Drawing for the job (mm, zero at the part's lowest x, y, z). Coordinates: 2 decimals unless noted, no trailing zeros. Order: outer loops, then holes, each group sorted by start corner. A loop starts at its lowest first (then second) coordinate and runs counter-clockwise, first axis right, second up. Notation, with made-up numbers: M -31.75,-36.5 L 16.25,-36.5 A26 ccw 16.25,-0.5 Z; hole C 54.5,17.25 d5. An arc over 180 degrees is marked long. Write item = value, one per line. Start each with the question number.
Q1. Band-saw the part on A-A on y = 7.5. Write the cut outline in (x, z), plus the area to 3 significant figures.
Q2. Drill centre lines: probe 1 along Y at (x, z) = (7.5, 1.35); probe 2 along Z at (x, y) = (13.25, 11.25); probe 3 along Y at (x, z) = (9, 3.75). Where is each one in solid material? Low to high.
Q3. Band-saw the part on C-C on z = 2.95. Write the cut outline in (x, y).
Q4. Pin check, flat tips, straight feed: P1, Ø1.5, axis at x = 6, z = 2, coming from the -Y side; P2, Ø2, axis at x = 9.5, z = 1.5, coming from the +Y side; P3, Ø2, axis at x = 12, z = 2.5, coming from the -Y side. Stop position of each tip, or through.
Q5. Pull direction X, two halves, no side cores. Call the marked faces 1, 2 and 3: released by +X, released by -X, zero draft, split by the parting line, or undercut.
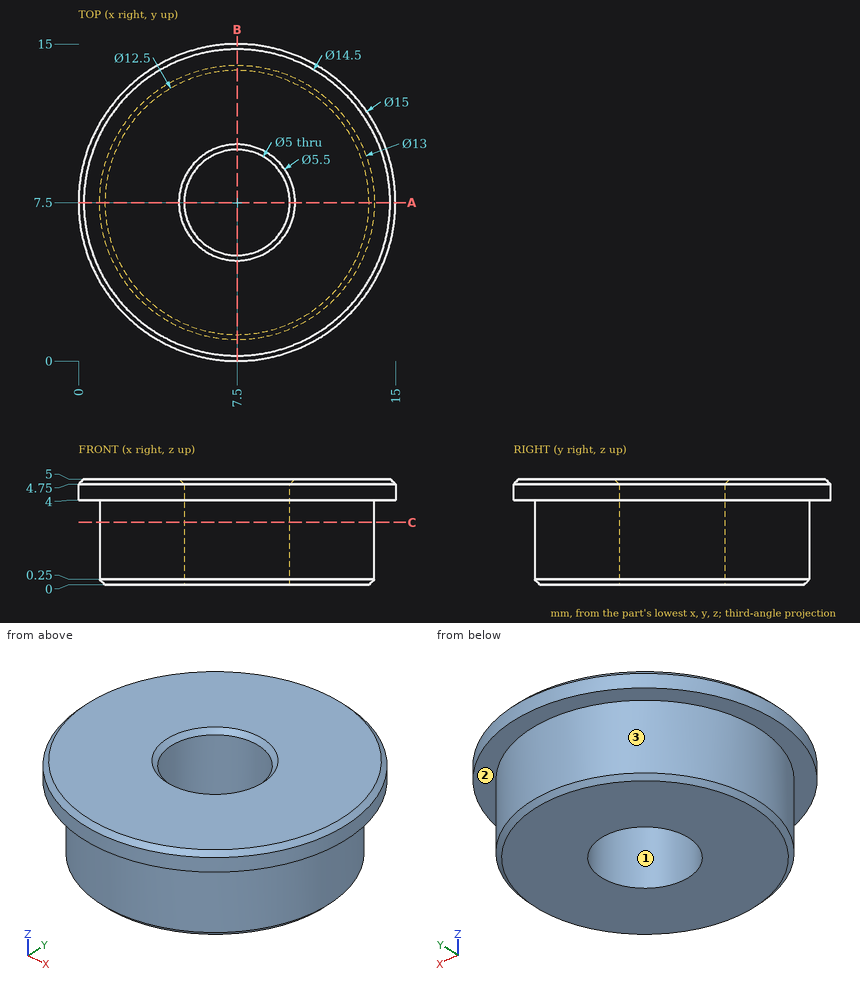
Recorded:
q1.outline = M 0,4 L 1,4 L 1,0.25 L 1.25,0 L 5,0 L 5,4.75 L 4.75,5 L 0.25,5 L 0,4.75 Z; M 10,0 L 13.75,0 L 14,0.25 L 14,4 L 15,4 L 15,4.75 L 14.75,5 L 10.25,5 L 10,4.75 Z
q1.area = 41.8 mm2
q2.probe_1 = 1 to 5, 10 to 14
q2.probe_2 = 4 to 5
q2.probe_3 = 1.18 to 5.5, 9.5 to 13.82
q3.outline = C 7.5,7.5 d13; hole C 7.5,7.5 d5
q4.P1 = 1.04
q4.P2 = 13.92
q4.P3 = 2.02
q5.face_1 = undercut
q5.face_2 = zero draft
q5.face_3 = split by the parting line
